from build123d import *

# Parameters (mm, degrees)
F1_DEPTH = 76.2
F2_R     = 12.7
F3_SCALE = 0.3


with BuildPart() as f1:
    # F0 (on Top) → F1 (new body)
    with BuildSketch(Plane.XY):
        Polygon((165.1, -95.25), (165.1, 95.25), (84.7781474317, 114.3), (69.85, 97.8762737351), (0, 97.8762737351), (-69.85, 97.8762737351), (-84.7781474317, 114.3), (-165.1, 95.25), (-165.1, -95.25), (-84.7781474317, -114.3), (-69.85, -97.8762737351), (0, -97.8762737351), (69.85, -97.8762737351), (84.7781474317, -114.3), align=None)
    extrude(amount=F1_DEPTH)

    # F2
    f2_edges = [f1.edges().sort_by_distance(p)[0] for p in [
        (-165.1, -95.25, 38.1),
        (-84.778147, -114.3, 38.1),
        (-69.85, -97.876274, 38.1),
        (69.85, -97.876274, 38.1),
        (84.778147, -114.3, 38.1),
        (165.1, -95.25, 38.1),
        (165.1, 95.25, 38.1),
        (84.778147, 114.3, 38.1),
        (69.85, 97.876274, 38.1),
        (-69.85, 97.876274, 38.1),
        (-84.778147, 114.3, 38.1),
        (-165.1, 95.25, 38.1),
    ]]
    fillet(f2_edges, radius=F2_R)


with BuildPart() as f1_1:
    # F3: moved
    add(f1.part.scale(F3_SCALE))


solid = f1_1.part
For this review, take the finished solid that the model builds, in its own axes (mm). A direction names the side the tool comes from. Round coordinates to 2 decimals unless told otherwise and drop trailing zeros. Loops run counter-clockwise (first coordinate to the right, second up) from the corner with the lowest first, then second, coordinate; pieces in that order, holes last. Notation, with made-up numbers: (87, 59.5) - (105, 59.5) arc R34 cw to (105, 98.5) - close; hole circle Ø3 at (-16, 81.25). An arc over 180 degrees is marked (long way). Answer as CSV lines item,"result".
(1) Consider section A-A on z = 18.5. Give the boundary of the cut face in (x, y).
Checked values:
outline,"(-49.53, -25.56) arc R3.81 ccw to (-46.6, -29.27) - (-27.62, -33.77) arc R3.81 ccw to (-23.92, -32.63) - (-22.09, -30.61) arc R3.81 cw to (-19.27, -29.36) - (19.27, -29.36) arc R3.81 cw to (22.09, -30.61) - (23.92, -32.63) arc R3.81 ccw to (27.62, -33.77) - (46.6, -29.27) arc R3.81 ccw to (49.53, -25.56) - (49.53, 25.56) arc R3.81 ccw to (46.6, 29.27) - (27.62, 33.77) arc R3.81 ccw to (23.92, 32.63) - (22.09, 30.61) arc R3.81 cw to (19.27, 29.36) - (-19.27, 29.36) arc R3.81 cw to (-22.09, 30.61) - (-23.92, 32.63) arc R3.81 ccw to (-27.62, 33.77) - (-46.6, 29.27) arc R3.81 ccw to (-49.53, 25.56) - close"
(2) Tool access review of faces 1 (the face through (-20.831, -29.698, 11.59)), 2 (the face through (23.018, 31.633, 11.27)), 3 (the face through (-1, 0, 22.86)): name each direction out of +Z, -Z, +X, -X, +Y, -Y from which nothing blocks a thin tool from reaching the whole face with its end or side.
Checked values:
face 1,"+Z, -Z, -Y"
face 2,"+Z, -Z, +Y"
face 3,"+Z, +X, -X, +Y, -Y"
(3) Mouldability with a two-part tool opening along X and no side actions: class faces 4 (the face through (-36.98, 31.55, 11.27)), 5 (the face through (-25.6, 33.7, 11.6)), 6 (the face through (25.6, 33.7, 11.6)), 7 (the face through (36.98, -31.55, 11.27)) as +X half, -X half, draft (parallel to the pull), parting line (faces both ways), or undercut.
Checked values:
face 4,"-X half"
face 5,"undercut"
face 6,"undercut"
face 7,"+X half"
(4) Consider section C-C on x = -32. Give the boundary of the cut face in (y, z), then the cut area to 3 significant figures.
Checked values:
outline,"(-32.73, 0) - (32.73, 0) - (32.73, 22.86) - (-32.73, 22.86) - close"
area,"1,500 mm2"
(5) Wall thickness on line 1 (Y direction, x = 4, z = 3.5); line 2 (Y direction, x = 41, z = 18.5); line 3 (X direction, y = -27, z = 19): over which ranges is each line inside the solid? List them lowest first.
Checked values:
line 1,"y = -29.36 to 29.36"
line 2,"y = -30.6 to 30.6"
line 3,"x = -49.25 to 49.25"
(6) Consider section B-B on x = -11. Give the boundary of the cut face in (y, z), then the cut area to 3 significant figures.
Checked values:
outline,"(-29.36, 0) - (29.36, 0) - (29.36, 22.86) - (-29.36, 22.86) - close"
area,"1,340 mm2"
(7) Insertion check: P1, Ø6, axis at x = 27, z = 12.5, coming from the -Y side; P2, Ø11.5, axis at x = -5, z = 6, coming from the +Y side; P3, Ø1, axis at x = 32.5, z = 13.5, coming from the +Y side; P4, Ø3, axis at x = 37, z = 15, coming from the +Y side. Each pin has a flat end and moves straight along its axis. Give the tip position at first contact, or say it passes through.
Checked values:
P1,"stops at y = -33.87"
P2,"stops at y = 29.36"
P3,"stops at y = 32.73"
P4,"stops at y = 31.9"
